For this review, take the finished solid that the model builds, in its own axes (mm). Round coordinates to 2 decimals unless told otherwise and drop trailing zeros. Write each loop counter-clockwise with the first axis right and the second up, starting at its lowest first coordinate (ties: lowest second). Pieces come first, ordered by that corner, then holes. Notation, with made-up numbers: (71, 64.5) -> (90, 64.5) arc R20 cw to (90, 79.5) -> close; hole circle Ø1 at (22, 27). An arc over 180 degrees is marked (long way). Answer as CSV lines item,"result". Start each with the question number.
Item 1: Wall thickness on probe 1 along Y at (x, z) = (2.2, -26); probe 2 along Y at (x, z) = (0.5, -28); probe 3 along Y at (x, z) = (2.55, -15.5): over which ranges is each line inside the solid? List them lowest first. Write a range as from..to.
Item 2: Take a section at B-B on z = -10. Give the boundary of the cut face in (x, y), then the cut area to 3 significant figures.
Item 3: For pin 1 Ø0.9 at (x, z) = (2, 7.5) entering from -Y; pin 2 Ø1.5 at (x, y) = (2, 24.5) entering from +Z, all flat-tipped, find the tip position at first contact; note any pin that passes through.
Item 4: Take a section at A-A on x = 0.8. Count the separate pieces of the cut face and the enclosed holes in it, then the cut area to 3 significant figures.
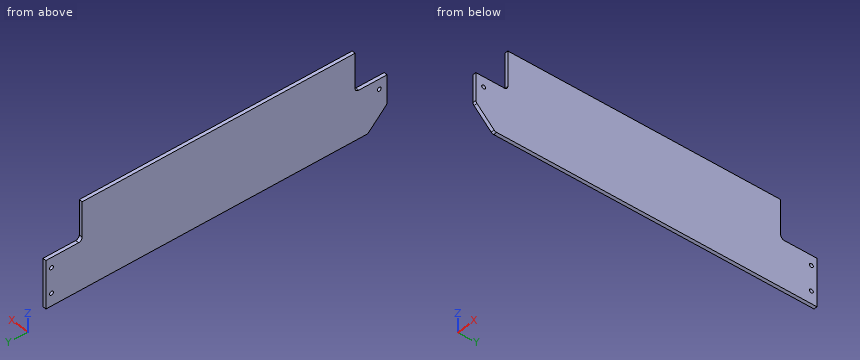
```python
from build123d import *

# Parameters (mm, degrees)
SKETCH1_R           = 1.65
BOSS_EXTRUDE1_DEPTH = 3
FILLET1_R           = 3.175


with BuildPart() as part:
    # Sketch1 → Boss-Extrude1 (new body)
    with BuildSketch(Plane(origin=(0, 0, 0), x_dir=(0, 0, -1), z_dir=(1, 0, 0))):
        Polygon((-15.875, 0), (18.0975, 0), (18.0975, 31.75), (60.325, 31.75), (60.325, -249.8725), (43.4975, -266.7), (18.0975, -266.7), (18.0975, -238.76), (-15.875, -238.76), align=None)
        with Locations((26.9875, 26.8732)):
            Circle(SKETCH1_R, mode=Mode.SUBTRACT)
        with Locations((49.2125, 26.8732)):
            Circle(SKETCH1_R, mode=Mode.SUBTRACT)
        with Locations(Location((26.9875, -259.9563, 0), (0, 0, 180))):
            Circle(SKETCH1_R, mode=Mode.SUBTRACT)
    extrude(amount=BOSS_EXTRUDE1_DEPTH)

    # Fillet1
    fillet1_edges = [part.edges().sort_by_distance(p)[0] for p in [
        (1.5, 0, -18.0975),
        (1.5, -249.8725, -60.325),
        (1.5, -266.7, -43.4975),
        (1.5, -238.76, -18.0975),
    ]]
    fillet(fillet1_edges, radius=FILLET1_R)


solid = part.part
```
Output values:
1,probe 1,"y = -266.7..-261.28, -258.63..25.55, 28.2..31.75"
1,probe 2,"y = -266.7..-261.26, -258.65..25.57, 28.18..31.75"
1,probe 3,"y = -238.81..0.05"
2,outline,"(0, -238.76) -> (3, -238.76) -> (3, 0) -> (0, 0) -> close"
2,area,"716 mm^2"
3,pin 1,"stops at y = -238.76"
3,pin 2,"stops at z = -18.1"
4,separate pieces,"1"
4,enclosed holes,"3"
4,area,"20,600 mm^2"
